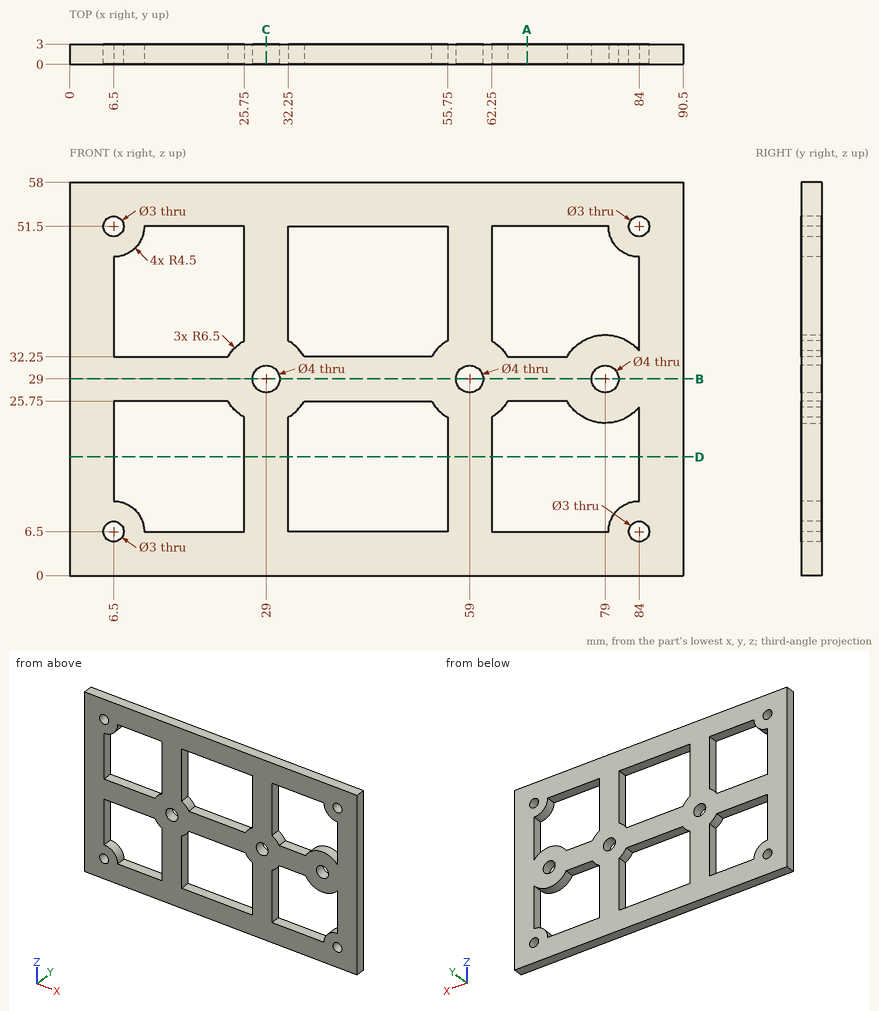
Part print with two shaded views. Sizes in mm from the minimum x, y, z corner. Coordinates: 2 decimals unless noted, no trailing zeros. Write each loop counter-clockwise with the first axis right and the second up, starting at its lowest first coordinate (ties: lowest second). Pieces come first, ordered by that corner, then holes. Notation, with made-up numbers: (54.25, -34.75) -> (85.25, -34.75) arc R21 cw to (85.25, -22.75) -> close; hole circle Ø3 at (6.5, 37). An arc over 180 degrees is marked (long way). Return JSON: item names as keys, results as strings. Group by question number.
Q1. Cut at C-C, the plane x = 29. Give the cut face in (y, z), then the cut area to 3 significant figures.
Q2. Cut at D-D, the plane z = 17.5. Give the cut face in (x, y).
Q3. Cut at B-B, the plane z = 29. Give the cut face in (x, y).
Q4. Cut at A-A, the plane x = 67.5. Give the cut face in (y, z), then the cut area to 3 significant figures.
Q5. Flat gauge pin, fed straight in: pin 1 (2.5 mm diameter, centred on x = 84, z = 51.5, fed in from +Y). Where does the tip first touch, or does it go through?
Q6. Drill centre lines: line 1 (X direction, y = 0.7, z = 29); line 2 (Z direction, x = 39, y = 2.8); line 3 (X direction, y = 0.55, z = 14.5). Where is each one in solid material? Low to high.
Returned:
{
 "1": {"outline": "(0, 0) -> (3, 0) -> (3, 27) -> (0, 27) -> close; (0, 31) -> (3, 31) -> (3, 58) -> (0, 58) -> close", "area": "162 mm2"},
 "2": {"outline": "(0, 0) -> (6.5, 0) -> (6.5, 3) -> (0, 3) -> close; (25.75, 0) -> (32.25, 0) -> (32.25, 3) -> (25.75, 3) -> close; (55.75, 0) -> (62.25, 0) -> (62.25, 3) -> (55.75, 3) -> close; (84, 0) -> (90.5, 0) -> (90.5, 3) -> (84, 3) -> close"},
 "3": {"outline": "(0, 0) -> (27, 0) -> (27, 3) -> (0, 3) -> close; (31, 0) -> (57, 0) -> (57, 3) -> (31, 3) -> close; (61, 0) -> (77, 0) -> (77, 3) -> (61, 3) -> close; (81, 0) -> (90.5, 0) -> (90.5, 3) -> (81, 3) -> close"},
 "4": {"outline": "(0, 0) -> (3, 0) -> (3, 6.5) -> (0, 6.5) -> close; (0, 25.75) -> (3, 25.75) -> (3, 32.25) -> (0, 32.25) -> close; (0, 51.5) -> (3, 51.5) -> (3, 58) -> (0, 58) -> close", "area": "58.5 mm2"},
 "5": {"pin 1": "passes through"},
 "6": {"line 1": "x = 0 to 27, 31 to 57, 61 to 77, 81 to 90.5", "line 2": "z = 0 to 6.5, 25.75 to 32.25, 51.5 to 58", "line 3": "x = 0 to 6.5, 25.75 to 32.25, 55.75 to 62.25, 84 to 90.5"}
}
